from build123d import *

# Parameters (mm, degrees)
ESQUISSE1_R        = 1.5
BOSS_EXTRU_1_DEPTH = 3


with BuildPart() as part:
    # Esquisse1 → Boss.-Extru.1 (new body)
    with BuildSketch(Plane.XY):
        with BuildLine():
            ThreePointArc((-27.380276014, -1.274350161), (-15.537335082, -7.194462147), (-2.33906069, -8.247329135))
            ThreePointArc((-2.33906069, -8.247329135), (5.804479886, -4.993281455), (11.147191658, 1.960962596))
            ThreePointArc((11.147191658, 1.960962596), (11.029757514, 4.289985461), (9.166322528, 5.692036935))
            ThreePointArc((9.166322528, 5.692036935), (6.013301366, 6.491366031), (2.936209941, 7.545869621))
            ThreePointArc((2.936209941, 7.545869621), (1.023768623, 8.032021848), (-0.949475558, 8.041142538))
            ThreePointArc((-0.949475558, 8.041142538), (-12.942714913, 6.878410061), (-24.974047874, 6.217528689))
            ThreePointArc((-24.974047874, 6.217528689), (-28.81213344, 3.317884658), (-27.380276014, -1.274350161))
        make_face()
        Circle(ESQUISSE1_R, mode=Mode.SUBTRACT)
        with Locations((8.6, 3)):
            Circle(ESQUISSE1_R, mode=Mode.SUBTRACT)
        with BuildLine():
            ThreePointArc((-25.549202237, 0.33835127), (-20.107029847, -2.924841196), (-14.056052845, -4.835689883))
            ThreePointArc((-14.056052845, -4.835689883), (-11.104571675, -4.479585719), (-8.90463517, -2.480003102))
            ThreePointArc((-8.90463517, -2.480003102), (-8.615705443, -0.657235742), (-8.90463517, 1.165531618))
            ThreePointArc((-8.90463517, 1.165531618), (-10.692993826, 3.307242171), (-13.334564289, 4.205716578))
            ThreePointArc((-13.334564289, 4.205716578), (-18.842020353, 4.354105802), (-24.349363894, 4.201597494))
            ThreePointArc((-24.349363894, 4.201597494), (-26.291680045, 2.686893023), (-25.549202237, 0.33835127))
        make_face(mode=Mode.SUBTRACT)
    extrude(amount=BOSS_EXTRU_1_DEPTH)


solid = part.part
Check sheet for the modelled part. Datum: model origin and axes. Units: mm. A direction names the side the tool comes from. Round coordinates to 2 decimals unless told otherwise and drop trailing zeros. Order: outer loops, then holes, each group sorted by start corner. A loop starts at its lowest first (then second) coordinate and runs counter-clockwise, first axis right, second up. Notation, with made-up numbers: M 10,36 L 42,36 A26 cw 42,52 Z; hole C -29,0 d6. An arc over 180 degrees is marked long. One line per item, written item: value. Start each with the question number.
1. Release check for a two-part mould opening along X. For faces 3 (the cylindrical face through (-28.79, 3.39, 1.48)), 4 (the cylindrical face through (-18.765, 4.354, 1.479)), 5 (the cylindrical face through (-1.5, 0.07, 1.48)), 6 (the cylindrical face through (11.045, 4.26, 1.479)) record: released by +X, released by -X, zero draft, split by the parting line, or undercut.
2. Scan lines: line 1 along X through (y, z) = (0.75, 2.4); line 2 along X through (y, z) = (-2.5, 0.3); line 3 along Y through (x, z) = (8.6, 1.2). Record each from-to range of solid material in increasing order.
3. Gauge pin test, flat ends, axial feed: P1, Ø1, axis at x = -19.5, z = 0.5, coming from the -Y side; P2, Ø1.8, axis at x = 8.6, y = 3, coming from the -Z side. Record the tip position at first contact, or that the pin passes through.
4. Section check C-C on x = -19.5. Enter the section's corners in (y, z).
5. Section check B-B on z = 2.4. Enter the section's corners in (x, y).
6. Section check D-D on y = -4. Enter the section's corners in (x, z).
7. Section check A-A on y = 3. Enter the section's corners in (x, z), and give its area (3 significant figures).
8. Access from +Z, -Z, +X, -X, +Y, -Y to the whole of each face (thin tool, end or side, straight path). Record for faces 1 (the cylindrical face through (6.057, 6.478, 1.479)), 2 (the cylindrical face through (-26.28, 2.72, 1.48)).
Results found:
1. face 3: released by -X
1. face 4: undercut
1. face 5: undercut
1. face 6: released by +X
2. line 1: -28.81 to -25.96, -8.79 to -1.3, 1.3 to 10.6
2. line 2: -25.68 to -21.01, -8.92 to 8.44
2. line 3: -2.31 to 1.5, 4.5 to 5.82
3. P1: y = -6.03
3. P2: through
4. outline: M -5.83,0 L -3.19,0 L -3.19,3 L -5.83,3 Z; M 4.35,0 L 6.46,0 L 6.46,3 L 4.35,3 Z
5. outline: M -27.38,-1.27 A34.7 ccw -2.34,-8.25 A16.57 ccw 11.15,1.96 A2.75 ccw 9.17,5.69 A39.74 cw 2.94,7.55 A8.1 ccw -0.95,8.04 A288.48 cw -24.97,6.22 A4.18 ccw Z; hole M -25.55,0.34 A27.15 ccw -14.06,-4.84 A4.89 ccw -8.9,-2.48 A5.89 ccw -8.9,1.17 A5.16 ccw -13.33,4.21 A100.88 ccw -24.35,4.2 A2.16 ccw Z; hole C 0,0 d3; hole C 8.6,3 d3
6. outline: M -23.26,0 L -17.32,0 L -17.32,3 L -23.26,3 Z; M -10.28,0 L 7,0 L 7,3 L -10.28,3 Z
7. outline: M -28.9,0 L -26.17,0 L -26.17,3 L -28.9,3 Z; M -10.29,0 L 7.1,0 L 7.1,3 L -10.29,3 Z; M 10.1,0 L 11.35,0 L 11.35,3 L 10.1,3 Z
7. area: 64.1 mm^2
8. face 1: +Z, -Z, +X, +Y
8. face 2: +Z, -Z
